from build123d import *

# Parameters (mm, degrees)
S_BOX1_W      = 51.8
S_BOX1_H      = 47.8
BOSS_1_DEPTH  = 4
S_CYL2_R      = 15
BOSS_2_DEPTH  = 8.1
S_BOX3_W      = 7.9
S_BOX3_H      = 28
BOSS_3_DEPTH  = 8.1
S_HOLE4_R     = 4
HOLE_4_DEPTH  = 12.2
S_HOLE5_R     = 3.5
HOLE_5_DEPTH  = 12.2
S_HOLE6_R     = 1.7
HOLE_6_DEPTH  = 12.2
S_HOLE7_R     = 1.7
HOLE_7_DEPTH  = 12.2
S_HOLE8_R     = 1.7
HOLE_8_DEPTH  = 12.2
S_HOLE9_R     = 1.7
HOLE_9_DEPTH  = 12.2
S_HOLE10_R    = 3.2
HOLE_10_DEPTH = 7.1
S_HOLE11_R    = 3.2
HOLE_11_DEPTH = 7.1
S_HOLE12_R    = 3.2
HOLE_12_DEPTH = 7.1
S_HOLE13_R    = 3.2
HOLE_13_DEPTH = 7.1
S_HOLE14_R    = 0.9
HOLE_14_DEPTH = 6.1
S_HOLE15_R    = 0.9
HOLE_15_DEPTH = 6.1


with BuildPart() as part:
    # S_box1 → Boss_1 (new body)
    with BuildSketch(Plane.XY):
        Rectangle(S_BOX1_W, S_BOX1_H)
    extrude(amount=BOSS_1_DEPTH)

    # S_cyl2 → Boss_2 (add)
    with BuildSketch(Plane.XY.offset(3.9)):
        Circle(S_CYL2_R)
    extrude(amount=BOSS_2_DEPTH)

    # S_box3 → Boss_3 (add)
    with BuildSketch(Plane.XY.offset(3.9)):
        with Locations((-21.95, 0)):
            Rectangle(S_BOX3_W, S_BOX3_H)
    extrude(amount=BOSS_3_DEPTH)

    # S_hole4 → Hole_4 (cut)
    with BuildSketch(Plane.XY.offset(-0.1)):
        with Locations(Location((-18, 0, 0), (0, 0, 270))):
            Circle(S_HOLE4_R)
    extrude(amount=HOLE_4_DEPTH, mode=Mode.SUBTRACT)

    # S_hole5 → Hole_5 (cut)
    with BuildSketch(Plane.XY.offset(-0.1)):
        Circle(S_HOLE5_R)
    extrude(amount=HOLE_5_DEPTH, mode=Mode.SUBTRACT)

    # S_hole6 → Hole_6 (cut)
    with BuildSketch(Plane.XY.offset(-0.1)):
        with Locations((7, 0)):
            Circle(S_HOLE6_R)
    extrude(amount=HOLE_6_DEPTH, mode=Mode.SUBTRACT)

    # S_hole7 → Hole_7 (cut)
    with BuildSketch(Plane.XY.offset(-0.1)):
        with Locations((0, 7)):
            Circle(S_HOLE7_R)
    extrude(amount=HOLE_7_DEPTH, mode=Mode.SUBTRACT)

    # S_hole8 → Hole_8 (cut)
    with BuildSketch(Plane.XY.offset(-0.1)):
        with Locations((-7, 0)):
            Circle(S_HOLE8_R)
    extrude(amount=HOLE_8_DEPTH, mode=Mode.SUBTRACT)

    # S_hole9 → Hole_9 (cut)
    with BuildSketch(Plane.XY.offset(-0.1)):
        with Locations((0, -7)):
            Circle(S_HOLE9_R)
    extrude(amount=HOLE_9_DEPTH, mode=Mode.SUBTRACT)

    # S_hole10 → Hole_10 (cut)
    with BuildSketch(Plane.XY.offset(5)):
        with Locations((7, 0)):
            Circle(S_HOLE10_R)
    extrude(amount=HOLE_10_DEPTH, mode=Mode.SUBTRACT)

    # S_hole11 → Hole_11 (cut)
    with BuildSketch(Plane.XY.offset(5)):
        with Locations((0, 7)):
            Circle(S_HOLE11_R)
    extrude(amount=HOLE_11_DEPTH, mode=Mode.SUBTRACT)

    # S_hole12 → Hole_12 (cut)
    with BuildSketch(Plane.XY.offset(5)):
        with Locations((-7, 0)):
            Circle(S_HOLE12_R)
    extrude(amount=HOLE_12_DEPTH, mode=Mode.SUBTRACT)

    # S_hole13 → Hole_13 (cut)
    with BuildSketch(Plane.XY.offset(5)):
        with Locations((0, -7)):
            Circle(S_HOLE13_R)
    extrude(amount=HOLE_13_DEPTH, mode=Mode.SUBTRACT)

    # S_hole14 → Hole_14 (cut)
    with BuildSketch(Plane(origin=(-26, 0, 0), x_dir=(0, 0, -1), z_dir=(1, 0, 0))):
        with Locations((-8, -10)):
            Circle(S_HOLE14_R)
    extrude(amount=HOLE_14_DEPTH, mode=Mode.SUBTRACT)

    # S_hole15 → Hole_15 (cut)
    with BuildSketch(Plane(origin=(-26, 0, 0), x_dir=(0, 0, -1), z_dir=(1, 0, 0))):
        with Locations((-8, 10)):
            Circle(S_HOLE15_R)
    extrude(amount=HOLE_15_DEPTH, mode=Mode.SUBTRACT)


solid = part.part
Source: CAD feature listing. Evaluate the final solid. Frame: model axes, mm. A direction names the side the tool comes from. Coordinates: 2 decimals unless noted, no trailing zeros. Order: outer loops, then holes, each group sorted by start corner. A loop starts at its lowest first (then second) coordinate and runs counter-clockwise, first axis right, second up. Notation, with made-up numbers: M 63,67.5 L 88,67.5 A12 ccw 88,82.5 Z; hole C 31,85 d11. An arc over 180 degrees is marked long. Write each question's results on one line, items separated by ' | '. Start each with the question number.
Item 1: Cut plane A-A (y = 0). Count the separate pieces of the cut face and the enclosed holes in it, and give its area (3 significant figures).
Item 2: First-contact query: pin 1 Ø4 at (x, y) = (0, 7) entering from +Z; pin 2 Ø10 at (x, y) = (18, 16.5) entering from -Z; pin 3 Ø0.5 at (y, z) = (-10.5, 8) entering from -X; pin 4 Ø7 at (x, y) = (-18, 0) entering from -Z. Flat tips, straight axial feed; report the tip coordinate or a pass-through.
Item 3: Line query: probe 1 along Y at (x, z) = (0, 2.05); probe 2 along Y at (x, z) = (-24.1, 8); probe 3 along Y at (x, z) = (0, 9.5). Output: solid intervals per line, ascending.
Item 4: Draft query along X for faces 4 (the face through (-0.417, -3.827, 8.451)), 5 (the face through (-19.9, 10, 8)), 6 (the face through (-23, 0, 12)). Return one class per face: pulls with the +X half, pulls with the -X half, needs draft (parallel to the pull), parting line crosses it, or undercut.
Item 5: Cut plane B-B (z = 7.75). Return loops of the section in (x, y).
Item 6: Cut plane D-D (y = 8). Return loops of the section in (x, z), and give its area (3 significant figures).
Item 7: Set-up query: faces 1 (the face through (5.65, -1.03, 2.46)), 2 (the face through (-22.94, -9.11, 8.12)), 3 (the face through (14.987, -0.626, 7.944)). Return all of +Z, -Z, +X, -X, +Y, -Y with unobstructed straight access to the full face (end or side cutting, diameter ignored); none if empty.
Item 8: Cut plane C-C (x = 7). Return loops of the section in (y, z).
Checked values:
1) separate pieces: 5 | enclosed holes: 0 | area: 231 mm2
2) pin 1: stops at z = 5 | pin 2: stops at z = 0 | pin 3: stops at x = -19.9 | pin 4: passes through
3) probe 1: y = -23.9 to -8.7, -5.3 to -3.5, 3.5 to 5.3, 8.7 to 23.9 | probe 2: y = -14 to -10.9, -9.1 to 9.1, 10.9 to 14 | probe 3: y = -15 to -10.2, -3.8 to -3.5, 3.5 to 3.8, 10.2 to 15
4) face 4: undercut | face 5: pulls with the -X half | face 6: needs draft
5) outline: M -25.9,-14 L -18,-14 L -18,-4 A4 cw -18,4 L -18,14 L -25.9,14 L -25.9,10.86 L -19.9,10.86 L -19.9,9.14 L -25.9,9.14 L -25.9,-9.14 L -19.9,-9.14 L -19.9,-10.86 L -25.9,-10.86 Z; M -14.81,-2.41 A15 ccw long -14.81,2.41 A4 cw Z; hole C -7,0 d6.4; hole C 0,0 d7; hole C 0,-7 d6.4; hole C 0,7 d6.4; hole C 7,0 d6.4
6) outline: M -25.9,0 L -1.37,0 L -1.37,5 L -3.04,5 L -3.04,12 L -12.69,12 L -12.69,4 L -18,4 L -18,12 L -25.9,12 Z; M 1.37,0 L 25.9,0 L 25.9,4 L 12.69,4 L 12.69,12 L 3.04,12 L 3.04,5 L 1.37,5 Z | area: 417 mm2
7) face 1: +Z, -Z | face 2: -X | face 3: +Z
8) outline: M -23.9,0 L -1.7,0 L -1.7,5 L -3.2,5 L -3.2,12 L -13.27,12 L -13.27,4 L -23.9,4 Z; M 1.7,0 L 23.9,0 L 23.9,4 L 13.27,4 L 13.27,12 L 3.2,12 L 3.2,5 L 1.7,5 Z
